CAD build for the part. Positions are in the model's coordinates, mm. Give positions to 0.01 mm unless a question says otherwise; leave off trailing zeros. Order: outer loops, then holes, each group sorted by start corner. A loop starts at its lowest first (then second) coordinate and runs counter-clockwise, first axis right, second up.
Solid Edge part; units mm, degrees
sketch "Sketch1" plane through (0, 0, 0) normal (0, 0, 1) x (1, 0, 0)
  circle A0 centre (0, 0) radius 3.175
extrude "Protrusion1" add sketch "Sketch1" along normal blind 63.5
chamfer "Chamfer1" distance 0.4762 angle 45 2 edges at (-3.175, 0, 0) (-3.175, 0, 63.5)
sketch "Sketch2" plane through (0, 0, 63.5) normal (0, 0, 1) x (1, 0, 0)
  line L0 (-0.9165, 1.5875) -> (0.9165, 1.5875)
  line L1 (1.8331, 0) -> (0.9165, 1.5875)
  line L2 (0.9165, -1.5875) -> (1.8331, 0)
  line L3 (-0.9165, -1.5875) -> (0.9165, -1.5875)
  line L4 (-1.8331, 0) -> (-0.9165, -1.5875)
  line L5 (-0.9165, 1.5875) -> (-1.8331, 0)
extrude "Cutout1" cut sketch "Sketch2" against normal blind 31.75
properties part number "162158"
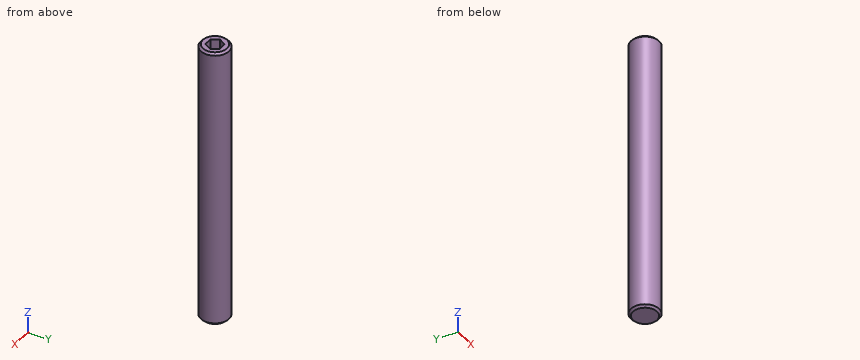
1. Wall check: line 1 (X direction, y = -1, z = 54); line 2 (X direction, y = 2.75, z = 5); line 3 (Z direction, x = -1.25, y = -0.5). Give the ranges that are in metal, low to high.
2. Saw through at C-C on z = 25. Give the cut face in (x, y) (3 decimals), plus the area to 3 significant figures.
3. Pin check, flat tips, straight feed: P1, Ø3, axis at y = 2.5, z = 54, coming from the +X side; P2, Ø1, axis at x = 0.5, y = 0, coming from the +Z side; P3, Ø1, axis at y = 1.5, z = 13.5, coming from the -X side. Stop position of each tip, or through.
Reported:
1. line 1: x = -3.01 to -1.26, 1.26 to 3.01
1. line 2: x = -1.59 to 1.59
1. line 3: z = 0 to 31.75
2. outline: circle Ø6.35 at (0, 0)
2. area: 31.7 mm2
3. P1: stops at x = 3.01
3. P2: stops at z = 31.75
3. P3: stops at x = -3.01
